from build123d import *
from build123d.topology import SkipClean

# Parameters (mm, degrees)
SKETCH1_R                                            = 60
SKETCH1_R_2                                          = 45
SKETCH1_R_3                                          = 40.00000000000001
BOSS_EXTRUDE3_DEPTH                                  = 10
SKETCH4_R                                            = 60.00000000000001
SKETCH4_R_2                                          = 50
BOSS_EXTRUDE4_DEPTH                                  = 6
SKETCH5_R                                            = 45.00000000000001
SKETCH5_R_2                                          = 42.5
BOSS_EXTRUDE5_DEPTH                                  = 8
FILLET1_R                                            = 2
SKETCH6_R                                            = 52.5
SKETCH6_R_2                                          = 42.500000000000014
CUT_EXTRUDE2_DEPTH                                   = 2
BOSS_EXTRUDE6_DEPTH                                  = 30
BOSS_EXTRUDE7_REACH                                  = 311.38
SKETCH8_R                                            = 20.5
CUT_EXTRUDE4_DEPTH                                   = 250.99199991039714
CUT_EXTRUDE4_DEPTH_BACK                              = 250.99199991039714
BOSS_EXTRUDE8_START                                  = 8
SKETCH9_R                                            = 15
BOSS_EXTRUDE8_DEPTH                                  = 8
SKETCH12_W                                           = 14.999999999999996
SKETCH12_H                                           = 15
BOSS_EXTRUDE9_DEPTH                                  = 25
CBORE_FOR_M3_HEXAGON_HEAD_BOLTS_FULL_THR_D           = 3.4
CBORE_FOR_M3_HEXAGON_HEAD_BOLTS_FULL_THR_CBORE_D     = 7
CBORE_FOR_M3_HEXAGON_HEAD_BOLTS_FULL_THR_CBORE_DEPTH = 2
CBORE_FOR_M3_HEXAGON_HEAD_BOLTS_FULL_2_D             = 3.4
CBORE_FOR_M3_HEXAGON_HEAD_BOLTS_FULL_2_CBORE_D       = 7
CBORE_FOR_M3_HEXAGON_HEAD_BOLTS_FULL_2_CBORE_DEPTH   = 2
SKETCH14_R                                           = 2.049999999999999
CUT_EXTRUDE5_DEPTH                                   = 15
SKETCH15_R                                           = 2.0499999999999985
CUT_EXTRUDE6_DEPTH                                   = 15
SKETCH16_R                                           = 6.000000000000016
CUT_EXTRUDE7_DEPTH                                   = 2.5
SKETCH17_R                                           = 6.000000000000003
CUT_EXTRUDE8_DEPTH                                   = 2.5


with BuildPart() as part:
    # Sketch1 → Boss-Extrude3 (new body)
    # profile 1 of 3: a face of its own
    with BuildSketch(Plane(origin=(0, 0, 0), x_dir=(0, 0, -1), z_dir=(1, 0, 0))):
        Circle(SKETCH1_R)
        Circle(SKETCH1_R_2, mode=Mode.SUBTRACT)
    # profile 2 of 3: a face of its own
    with BuildSketch(Plane(origin=(0, 0, 0), x_dir=(0, 0, -1), z_dir=(1, 0, 0))):
        with BuildLine():
            ThreePointArc((-23.076923076923066, 55.38461538461536), (-60.77677297236316, 43.883864861815795), (-100, 39.99999999999997))
            Line((-100, 39.999999999999986), (-200, 39.99999999999997))
            ThreePointArc((-200, 39.999999999999986), (-171.7157287525381, 28.284271247461877), (-160, -2.449e-14))
            ThreePointArc((-160, -3.429e-14), (-171.7157287525381, -28.284271247461938), (-200, -40.00000000000003))
            Line((-200, -40.00000000000003), (-100, -40.000000000000014))
            ThreePointArc((-100, -40.00000000000003), (-60.776772972363155, -43.88386486181582), (-23.07692307692308, -55.38461538461539))
            ThreePointArc((-23.0769230769231, -55.38461538461537), (-60, 7.35e-15), (-23.076923076923073, 55.38461538461539))
        make_face()
    # profile 3 of 3: a face of its own
    with BuildSketch(Plane(origin=(0, 0, 0), x_dir=(0, 0, -1), z_dir=(1, 0, 0))):
        with Locations((-200, -2.449e-14)):
            Circle(SKETCH1_R_3)
    extrude(amount=BOSS_EXTRUDE3_DEPTH)

    # Sketch4 → Boss-Extrude4 (add)
    with BuildSketch(Plane(origin=(10, 0, 0), x_dir=(0, 0, -1), z_dir=(1, 0, 0))):
        with Locations(Location((0, 0, 0), (0, 0, 112.619864948))):
            Circle(SKETCH4_R)
        Circle(SKETCH4_R_2, mode=Mode.SUBTRACT)
    extrude(amount=BOSS_EXTRUDE4_DEPTH)

    # Sketch5 → Boss-Extrude5 (add)
    with BuildSketch(Plane.ZY):
        with Locations(Location((0, 0, 0), (0, 0, 180))):
            Circle(SKETCH5_R)
        Circle(SKETCH5_R_2, mode=Mode.SUBTRACT)
    extrude(amount=-BOSS_EXTRUDE5_DEPTH)

    # Fillet1
    fillet1_edges = [part.edges().sort_by_distance(p)[0] for p in [
        (8, -1.102e-14, 45.00000000000001),
    ]]
    fillet(fillet1_edges, radius=FILLET1_R - 0.0001)  # a hair under: the kernel refuses the full size

    # Sketch6 → Cut-Extrude2 (cut)
    with BuildSketch(Plane.ZY):
        Circle(SKETCH6_R)
        Circle(SKETCH6_R_2, mode=Mode.SUBTRACT)
    extrude(amount=-CUT_EXTRUDE2_DEPTH, mode=Mode.SUBTRACT)

    # Sketch7 → Boss-Extrude6 (add)
    with BuildSketch(Plane(origin=(16, 0, 0), x_dir=(0, 0, -1), z_dir=(1, 0, 0))):
        with BuildLine():
            ThreePointArc((60.00000000000001, -1.2e-16), (42.42640687119286, 42.42640687119285), (7.35e-15, 60.000000000000014))
            Line((0, 60.00000000000001), (0, 52.000000000000014))
            ThreePointArc((5.5e-14, 52.000000000000014), (52, -2.872e-14), (-9.55e-15, -52))
            Line((0, -52), (0, -60.00000000000001))
            ThreePointArc((0, -60), (42.42640687119285, -42.42640687119285), (60.00000000000001, -1.2e-16))
        make_face()
    extrude(amount=BOSS_EXTRUDE6_DEPTH)

    # Sketch8 → Boss-Extrude7 (add, up to next)
    with BuildSketch(Plane(origin=(0, 0, -60), x_dir=(-1, 0, 0), z_dir=(0, 0, -1)), mode=Mode.PRIVATE) as boss_extrude7_sk1:
        with Locations((-25.500000000000004, -2.72e-15)):
            Circle(SKETCH8_R)
    boss_extrude7_tool1 = extrude(boss_extrude7_sk1.sketch, amount=-BOSS_EXTRUDE7_REACH, mode=Mode.PRIVATE) - part.part
    add(boss_extrude7_tool1.solids().sort_by_distance((25.5, 0, -60))[0])
    add(boss_extrude7_tool1.solids().sort_by_distance((25.5, 0, -60))[1])

    # Sketch11 → Cut-Extrude4 (cut, two sides: drawn at the far end of the back side and taken through both)
    with BuildSketch(Plane(origin=(10, 0, 0), x_dir=(0, 0, -1), z_dir=(1, 0, 0)).offset(-CUT_EXTRUDE4_DEPTH_BACK)):
        with BuildLine():
            Line((-200, 29.999999999999975), (-200, 39.99999999999997))
            ThreePointArc((-200, 39.99999999999997), (-240, -1.959e-14), (-200, -40.00000000000003))
            Line((-200, -40.00000000000003), (-200, -30.000000000000025))
            ThreePointArc((-200, -30.000000000000025), (-230, -2.082e-14), (-200, 29.999999999999975))
        make_face()
    extrude(amount=CUT_EXTRUDE4_DEPTH + CUT_EXTRUDE4_DEPTH_BACK, mode=Mode.SUBTRACT)

    # Sketch9 → Boss-Extrude8 (add)
    with SkipClean():  # the faces are left unmerged after this step: merging them gives an invalid solid
        with BuildSketch(Plane(origin=(0, 0, -60), x_dir=(-1, 0, 0), z_dir=(0, 0, -1)).offset(BOSS_EXTRUDE8_START)):
            with BuildLine():
                ThreePointArc((-5.000000000000001, 0), (-25.500000000000007, 20.5), (-46, 0))
                ThreePointArc((-46, 0), (-25.500000000000007, -20.5), (-5.000000000000001, 0))
            make_face()
            with Locations((-25.500000000000004, -2.72e-15)):
                Circle(SKETCH9_R, mode=Mode.SUBTRACT)
        extrude(amount=-BOSS_EXTRUDE8_DEPTH)

    # Sketch12 → Boss-Extrude9 (add)
    with SkipClean():  # the faces are left unmerged after this step: merging them gives an invalid solid
        with BuildSketch(Plane(origin=(0, 0, -60), x_dir=(-1, 0, 0), z_dir=(0, 0, -1))):
            with Locations((-25.5, -3.11e-15)):
                Rectangle(SKETCH12_W, SKETCH12_H)
        extrude(amount=BOSS_EXTRUDE9_DEPTH)

    # CBORE for M3 Hexagon head bolts-Full thread-grades AB1 (through all)
    with Locations(Plane(origin=(41, -54.543560573, -25), x_dir=(0, 0.416666666667, -0.909059342886), z_dir=(0, -0.909059342886, -0.416666666667))):
        with Locations((0, 0)):
            CounterBoreHole(CBORE_FOR_M3_HEXAGON_HEAD_BOLTS_FULL_THR_D / 2, CBORE_FOR_M3_HEXAGON_HEAD_BOLTS_FULL_THR_CBORE_D / 2, CBORE_FOR_M3_HEXAGON_HEAD_BOLTS_FULL_THR_CBORE_DEPTH)

    # CBORE for M3 Hexagon head bolts-Full 2 (through all)
    with Locations(Plane(origin=(41, 54.543560573, -25), x_dir=(0, 0.416667072006, 0.909059157099), z_dir=(0, 0.909059157099, -0.416667072006))):
        with Locations((0, 0)):
            CounterBoreHole(CBORE_FOR_M3_HEXAGON_HEAD_BOLTS_FULL_2_D / 2, CBORE_FOR_M3_HEXAGON_HEAD_BOLTS_FULL_2_CBORE_D / 2, CBORE_FOR_M3_HEXAGON_HEAD_BOLTS_FULL_2_CBORE_DEPTH)

    # Sketch14 → Cut-Extrude5 (cut)
    with SkipClean():  # the faces are left unmerged after this step: merging them gives an invalid solid
        with BuildSketch(Plane(origin=(0, 119.51150572225207, 68.9999999999988), x_dir=(1, 0, 0), z_dir=(0, 0.8660254037844414, 0.49999999999999517))):
            with Locations(Location((4.999999999999994, -173.20508075688855, 0), (0, 0, 270))):
                Circle(SKETCH14_R)
        extrude(amount=-CUT_EXTRUDE5_DEPTH, mode=Mode.SUBTRACT)

    # Sketch15 → Cut-Extrude6 (cut)
    with SkipClean():  # the faces are left unmerged after this step: merging them gives an invalid solid
        with BuildSketch(Plane(origin=(0, -119.5115057222521, 68.99999999999882), x_dir=(-1, 0, 0), z_dir=(0, -0.8660254037844414, 0.49999999999999517))):
            with Locations(Location((-4.999999999999994, -173.20508075688852, 0), (0, 0, 90))):
                Circle(SKETCH15_R)
        extrude(amount=-CUT_EXTRUDE6_DEPTH, mode=Mode.SUBTRACT)

    # Sketch16 → Cut-Extrude7 (cut)
    with SkipClean():  # the faces are left unmerged after this step: merging them gives an invalid solid
        with BuildSketch(Plane(origin=(10, 0, 0), x_dir=(0, 0, -1), z_dir=(1, 0, 0))):
            with Locations((-200, 0)):
                Circle(SKETCH16_R)
        extrude(amount=-CUT_EXTRUDE7_DEPTH, mode=Mode.SUBTRACT)

    # Sketch17 → Cut-Extrude8 (cut)
    with SkipClean():  # the faces are left unmerged after this step: merging them gives an invalid solid
        with BuildSketch(Plane(origin=(10, 0, 0), x_dir=(0, 0, -1), z_dir=(1, 0, 0))):
            with Locations((-80, -25)):
                Circle(SKETCH17_R)
            with Locations((-80, 25)):
                Circle(SKETCH17_R)
        extrude(amount=-CUT_EXTRUDE8_DEPTH, mode=Mode.SUBTRACT)


solid = part.part
Check sheet for the modelled part. Datum: model origin and axes. Units: mm. A direction names the side the tool comes from. Round coordinates to 2 decimals unless told otherwise and drop trailing zeros. Loops run counter-clockwise (first coordinate to the right, second up) from the corner with the lowest first, then second, coordinate; pieces in that order, holes last. Notation, with made-up numbers: M 33.25,79 L 65.25,79 A22 ccw 65.25,110 Z; hole C 41.5,-1 d1. An arc over 180 degrees is marked long. One line per item, written item: value.
(1) Sectioned sample at D-D, the plane z = 127.5. Record the cut outline in (x, y).
Computed values:
outline: M 0,-40 L 10,-40 L 10,40 L 0,40 Z
(2) Release check for a two-part mould opening along X. For faces 6 (the face through (26, 7.5, -72)), 7 (the face through (2, 0, 43)), 8 (the face through (5, 40, 149)) record: +X half, -X half, draft (parallel to the pull), parting line (faces both ways), or undercut.
Computed values:
face 6: undercut
face 7: -X half
face 8: draft
(3) Sectioned sample at C-C, the plane z = 80. Record the cut outline in (x, y), then the cut area to 3 significant figures.
Computed values:
outline: M 0,-41 L 10,-41 L 10,-31 L 7.5,-31 L 7.5,-19 L 10,-19 L 10,19 L 7.5,19 L 7.5,31 L 10,31 L 10,41 L 0,41 Z
area: 760 mm^2
(4) Depth check by flat-ended pin: pin 1 Ø4.5 at (y, z) = (3, -78) entering from +X; pin 2 Ø14 at (y, z) = (-25, 80) entering from -X; pin 3 Ø8 at (x, z) = (6, 169) entering from +Y; pin 4 Ø3 at (x, y) = (6.5, 36.5) entering from +Z. Enter the tip coordinate at first touch or a pass-through.
Computed values:
pin 1: stops at x = 33
pin 2: stops at x = 0
pin 3: stops at y = 40
pin 4: stops at z = 200
(5) Thickness scan on line 1 (Y direction, x = 25, z = -65); line 2 (Y direction, x = 10.05, z = 0); line 3 (Z direction, x = 15, y = -30). Record the ranges inside material, lowest first.
Computed values:
line 1: y = -20.49 to -14.99, -7.5 to 7.5, 14.99 to 20.49
line 2: y = -60 to -50, 50 to 60
line 3: z = -51.96 to -40, 40 to 51.96
(6) Access from +Z, -Z, +X, -X, +Y, -Y to the whole of each face (thin tool, end or side, straight path). Record for faces 1 (the face through (30.79, 1.143, -51.987)), 2 (the face through (7.5, -25, 80)), 3 (the face through (40.485, 0.66, -64.056)), 4 (the face through (31, -56, 0)), 5 (the face through (5, -40, 151)).
Computed values:
face 1: +Z, +X
face 2: +X
face 3: -Z
face 4: +Z, +X, +Y, -Y
face 5: +Z, +X, -X, -Y
(7) Sectioned sample at B-B, the plane x = 25.5. Record the cut outline in (y, z).
Computed values:
outline: M -60,0 A60 ccw -20.5,-56.39 L -20.5,-68 L -15,-68 L -15,-60 L -7.5,-60 L -7.5,-85 L 7.5,-85 L 7.5,-60 L 15,-60 L 15,-68 L 20.5,-68 L 20.5,-56.39 A60 ccw 60,0 L 52,0 A52 cw -52,0 Z
(8) Sectioned sample at A-A, the plane z = 197. Record the cut outline in (x, y).
Computed values:
outline: M 0,-40 L 10,-40 L 10,-5.2 L 7.5,-5.2 L 7.5,5.2 L 10,5.2 L 10,40 L 0,40 Z
